Geometry: see drawing. Coordinates: mm, zero at the bounding-box minimum. A direction names the side the tool comes from. Coordinates: 2 decimals unless noted, no trailing zeros. Loops run counter-clockwise (first coordinate to the right, second up) from the corner with the lowest first, then second, coordinate; pieces in that order, holes last. Notation, with made-up numbers: (-36.75, 36.25) -> (19.25, 36.25) arc R19 cw to (19.25, 68.25) -> close; hole circle Ø10 at (-8, 11.5). An arc over 180 degrees is marked (long way). Put each result on its own line as item: value. Start each with the question number.
1) Cut plane C-C (z = 13). Return the cut outline in (x, y).
2) Material intervals for L1, parallel to Y at x = 63, z = 45; L2, parallel to Y at x = 10, z = 69; L3, parallel to Z at x = 35, y = 58, sorted ascending.
3) Cut plane D-D (y = 58). Return the cut outline in (x, z).
4) Cut plane B-B (z = 66.5). Return the cut outline in (x, y), plus the area to 4 significant figures.
5) Pull-direction query (X, two-part tool) for the marked faces 5, 6, 7 and 8; classes: pulls with the +X half, pulls with the -X half, needs draft (parallel to the pull), parting line crosses it, or undercut.
6) Set-up query: the marked faces 1, 2, 3 and 4. Return all of +Z, -Z, +X, -X, +Y, -Y with unobstructed straight access to the full face (end or side cutting, diameter ignored); none if empty.
7) Contact query for flat-ended pins moving along their axis: P1, Ø6, axis at y = 45, z = 22, coming from the -X side; P2, Ø22.5, axis at x = 70.5, y = 39.5, coming from the +Z side; P3, Ø24, axis at y = 9, z = 31, coming from the -X side. Output: stop coordinate, or through.
8) Cut plane A-A (y = 38). Return the cut outline in (x, z).
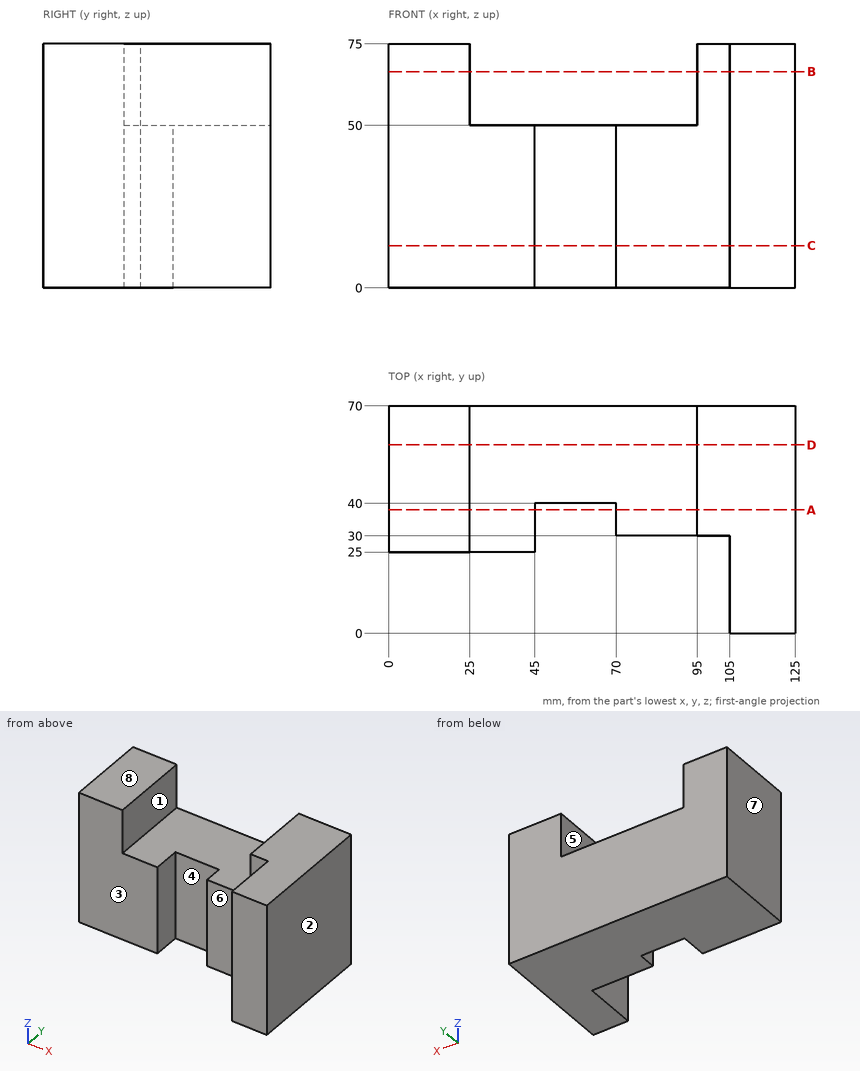
Results found:
1. outline: (0, 25) -> (45, 25) -> (45, 40) -> (70, 40) -> (70, 30) -> (105, 30) -> (105, 0) -> (125, 0) -> (125, 70) -> (0, 70) -> close
2. L1: y = 40 to 70
2. L2: y = 25 to 70
2. L3: z = 0 to 50
3. outline: (0, 0) -> (125, 0) -> (125, 75) -> (95, 75) -> (95, 50) -> (25, 50) -> (25, 75) -> (0, 75) -> close
4. outline: (0, 25) -> (25, 25) -> (25, 70) -> (0, 70) -> close; (95, 30) -> (105, 30) -> (105, 0) -> (125, 0) -> (125, 70) -> (95, 70) -> close
4. area: 2,925 mm2
5. face 5: undercut
5. face 6: undercut
5. face 7: pulls with the -X half
5. face 8: needs draft
6. face 1: +Z, +Y, -Y
6. face 2: +Z, -Z, +X, +Y, -Y
6. face 3: +Z, -Z, -X, -Y
6. face 4: +Z, -Z, -Y
7. P1: stops at x = 0
7. P2: stops at z = 50
7. P3: stops at x = 105
8. outline: (0, 0) -> (45, 0) -> (45, 50) -> (25, 50) -> (25, 75) -> (0, 75) -> close; (70, 0) -> (125, 0) -> (125, 75) -> (95, 75) -> (95, 50) -> (70, 50) -> close
